from build123d import *

# Parameters (mm, degrees)
F3_D     = 7.6
F3_DEPTH = 12
F3_TIP   = 2.2832703523
F5_D     = 7.6
F5_DEPTH = 12
F5_TIP   = 2.2832703523


with BuildPart() as f1:
    # F0 (on Front) → F1 (revolve)
    with BuildSketch(Plane.XZ):
        Polygon((-18, -30.0000015049), (-30, -48.0000015049), (0, -48.0000015049), (0, 0), (-27, 0), align=None)
    revolve(axis=Axis((0, 0, -24.0000007525), (0, 0, -1)))

    # F3
    with Locations(Plane.XY):
        with Locations((4.7843093053, 16.9646441936), (0, 3.9457264356), (16.4348743856, 5.9969499707), (-9.1730067506, 16.7864412069), (7.7405036427, -11.5405060351), (-6.8799313158, -12.1632143855), (-18.984535709, -2.4492875673)):
            Hole(F3_D / 2, depth=F3_DEPTH)
            with Locations((0, 0, -(F3_DEPTH + F3_TIP / 2))):  # 118° drill point
                Cone(0, F3_D / 2, F3_TIP, mode=Mode.SUBTRACT)

    # F5
    with Locations(Plane.XY):
        with Locations((-13.827174902, 7.3514520191), (1.784414053, -19.2592125386), (16.5089797229, -4.1798353195)):
            Hole(F5_D / 2, depth=F5_DEPTH)
            with Locations((0, 0, -(F5_DEPTH + F5_TIP / 2))):  # 118° drill point
                Cone(0, F5_D / 2, F5_TIP, mode=Mode.SUBTRACT)


solid = f1.part
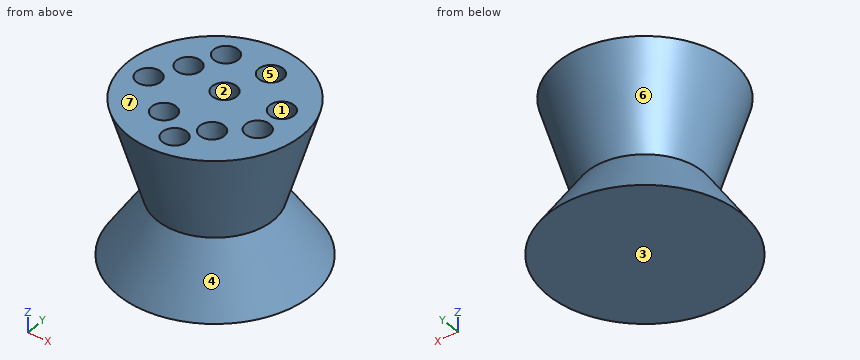
Can you work these out from the model? Positions are in its coordinate system, mm. Face numbers are marked on the shaded views. A direction names the side the tool comes from. Give positions to 0.01 mm unless a question says otherwise; leave off trailing zeros. Write each loop counter-clockwise with the first axis right and the second up, starting at its lowest first coordinate (ties: lowest second). Pieces come first, ordered by that corner, then holes. Notation, with made-up numbers: (58, 41.5) -> (83, 41.5) arc R18 cw to (83, 76.5) -> close; hole circle Ø2 at (25, 85). An arc over 180 degrees is marked (long way). Answer as a JSON object with one key per item and string values. Group by question number.
Item 1: I'm going to push flat-ended pins straight in: P1, Ø1, axis at x = -4.5, z = -11, coming from the -Y side; P2, Ø5, axis at x = -12.5, z = -33.5, coming from the -Y side; P3, Ø1.5, axis at y = -15, z = -41, coming from the +X side. Where does each tip first touch, or does it pass through?
Item 2: Suppose I cut it at B-B (z = -24). Please give me the cut outline in (x, y).
Item 3: We'd pull the mould along Y, two halves only. Please class the marked faces 1, 2, 3 and 4: +Y half, -Y half, draft (parallel to the pull), parting line (faces both ways), or undercut.
Item 4: Suppose I cut it at A-A (z = -6.5). State how many separate pieces and enclosed holes the cut face has, plus the area to 3 significant figures.
Item 5: Please list where these lines run through material, in increasing order: line 1 (X direction, y = -3.5, z = -3); line 2 (X direction, y = 9, z = -7.5); line 3 (Z direction, x = 15, y = 15.5). Write a range as [from, to].
Item 6: For the marked faces 5, 6 and 7, which set-ups out of +Z, -Z, +X, -X, +Y, -Y let a thin tool reach every point of the face, with its end or its side?
Findings:
{
 "1": {"P1": "stops at y = -23.45", "P2": "stops at y = -18.67", "P3": "stops at x = 21.23"},
 "2": {"outline": "circle Ø39.6 at (0, 0)"},
 "3": {"face 1": "undercut", "face 2": "undercut", "face 3": "draft", "face 4": "parting line"},
 "4": {"separate pieces": "1", "enclosed holes": "10", "area": "1,520 mm²"},
 "5": {"line 1": "x = [-25.86, -22.64], [-15.33, 12.77], [20.25, 25.86]", "line 2": "x = [-23.06, -17.25], [-10.4, 14.11], [18.76, 23.06]", "line 3": "z = [-48, -35.35], [-18.1, 0]"},
 "6": {"face 5": "+Z", "face 6": "none", "face 7": "+Z, +X, -X, +Y, -Y"}
}
